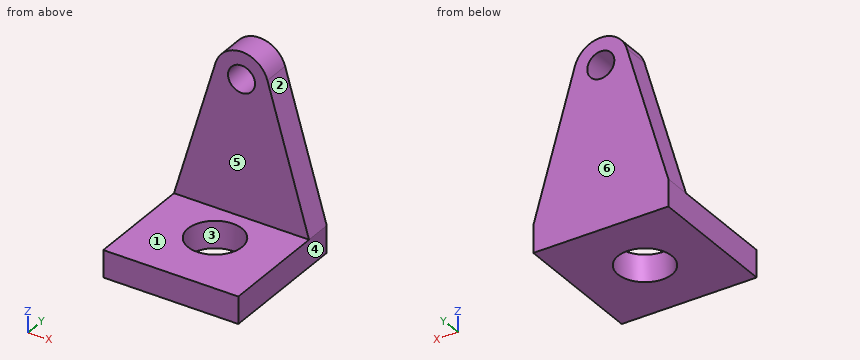
Autodesk Inventor part; units mm, degrees
ref_plane "Work Plane1" through (0, 25, 0) normal (0, 1, 0) x (-1, 0, 0)
ref_plane "YZ Plane" through (0, 0, 0) normal (1, 0, 0) x (0, 1, 0)
ref_plane "XY Plane" through (0, 0, 0) normal (0, 0, 1) x (1, 0, 0)
sketch "Sketch1" plane through (0, 0, 0) normal (0, 0, 1) x (1, 0, 0)
  line L0 (-335.2657, 170.906) -> (-144.554, 170.906) construction
  line L1 (-144.554, 170.906) -> (-144.554, -100.0273) construction
  line L2 (-144.554, -100.0273) -> (-335.2657, -100.0273) construction
  line L3 (-335.2657, -100.0273) -> (-335.2657, 170.906) construction
  line L4 (-25, 25) -> (25, 25)
  line L5 (25, 25) -> (25, -25)
  line L6 (25, -25) -> (-25, -25)
  line L7 (-25, -25) -> (-25, 25)
  line L8 (-25, 25) -> (25, -25) construction
  line L9 (25, 25) -> (-25, -25) construction
  circle A0 centre (0, 0) radius 10
  dimension "d6" = 50
  dimension "d7" = 50
  dimension "d8" = 20
extrude "Extrusion1" add sketch "Sketch1" along normal blind 10
ref_plane "Work Plane1" through (0, 25, 0) normal (0, 1, 0) x (-1, 0, 0)
sketch "Sketch2" plane through (-25, 25, 0) normal (0, 1, 0) x (1, 0, 0)
  arc A0 (15.4, -62.8) -> (34.6, -62.8) centre (25, -60) ccw
  circle A1 centre (25, -60) radius 5
  line L0 (50, -10) -> (0, -10)
  line L1 (50, -10) -> (34.6, -62.8)
  line L2 (0, -10) -> (15.4, -62.8)
  line L3 (0, -10) -> (50, -10)
  line L4 (50, -10) -> (0, -10)
  line L5 (0, -10) -> (50, -10)
  point P0 (25, 0)
  dimension "d13" = 20
  dimension "d14" = 10
  dimension "d15" = 50
extrude "Extrusion2" add sketch "Sketch2" against normal blind 10
properties part number "cad@35"
The model under review builds one solid part; all positions refer to its coordinate system, in mm. Face numbers are marked on the shaded views. A direction names the side the tool comes from. Coordinates: 2 decimals unless noted, no trailing zeros. Write each loop counter-clockwise with the first axis right and the second up, starting at its lowest first coordinate (ties: lowest second). Pieces come first, ordered by that corner, then holes. Notation, with made-up numbers: (-37.5, -19) -> (-3.5, -19) arc R29 ccw to (-3.5, 4) -> close; hole circle Ø8 at (-32.75, -0.5). An arc over 180 degrees is marked (long way). One line per item, written item: value. Start each with the question number.
Q1. Add section B-B, the plane y = 0. Give the boundary of the cut face in (x, z).
Q2. Add section D-D, the plane x = 7. Give the boundary of the cut face in (y, z).
Q3. To check wall thickness, follow probe 1 along Y at (x, z) = (0, 2.5); probe 2 along Z at (x, y) = (0, 21.25); probe 3 along Y at (x, z) = (-16, 24.5). State the ranges of each line that lie inside material, in increasing order.
Q4. The part is to be moulded in two halves that separate along Y. For the marked faces 3, 4, 5 and 6, say which applies: +Y half, -Y half, draft (parallel to the pull), parting line (faces both ways), or undercut.
Q5. For the marked faces 1 and 2, list the 3-axis set-ups (+Z, -Z, +X, -X, +Y, -Y) from which the entire face can be reached by the end or side of a thin tool; tool diameter is ignored.
Q6. Clearance check with flat-ended pins moving along their axes: P1, Ø8, axis at x = -2.5, z = 37.5, coming from the -Y side; P2, Ø2, axis at x = 14.5, y = -14.5, coming from the +Z side. State where each tip first meets the part, or that it passes through.
Q7. Add section C-C, the plane z = 60. Give the boundary of the cut face in (x, y).
Q8. Add section A-A, the plane x = 0. Give the boundary of the cut face in (y, z).
Response:
1. outline: (-25, 0) -> (-10, 0) -> (-10, 10) -> (-25, 10) -> close; (10, 0) -> (25, 0) -> (25, 10) -> (10, 10) -> close
2. outline: (-25, 0) -> (-7.14, 0) -> (-7.14, 10) -> (-25, 10) -> close; (7.14, 0) -> (25, 0) -> (25, 67.14) -> (15, 67.14) -> (15, 10) -> (7.14, 10) -> close
3. probe 1: -25 to -10, 10 to 25
3. probe 2: 0 to 55, 65 to 70
3. probe 3: 15 to 25
4. face 3: undercut
4. face 4: draft
4. face 5: -Y half
4. face 6: +Y half
5. face 1: +Z, +X, -X, -Y
5. face 2: +Z, +X, +Y, -Y
6. P1: y = 15
6. P2: z = 10
7. outline: (-10.42, 15) -> (-5, 15) -> (-5, 25) -> (-10.42, 25) -> close; (5, 15) -> (10.42, 15) -> (10.42, 25) -> (5, 25) -> close
8. outline: (-25, 0) -> (-10, 0) -> (-10, 10) -> (-25, 10) -> close; (10, 0) -> (25, 0) -> (25, 55) -> (15, 55) -> (15, 10) -> (10, 10) -> close; (15, 65) -> (25, 65) -> (25, 70) -> (15, 70) -> close
